Study the drawing (mm; zero at the part's minimum x, y, z) and answer. A direction names the side the tool comes from. Coordinates: 2 decimals unless noted, no trailing zeros. Order: outer loops, then holes, each group sorted by start corner. A loop starts at its lowest first (then second) coordinate and runs counter-clockwise, first axis right, second up. Notation, with made-up numbers: M 33.25,66 L 74.25,66 A12 ccw 74.25,79 Z; hole C 40,0 d9. An arc over 180 degrees is marked long. Use a Markdown table: item, result. Add a question column.
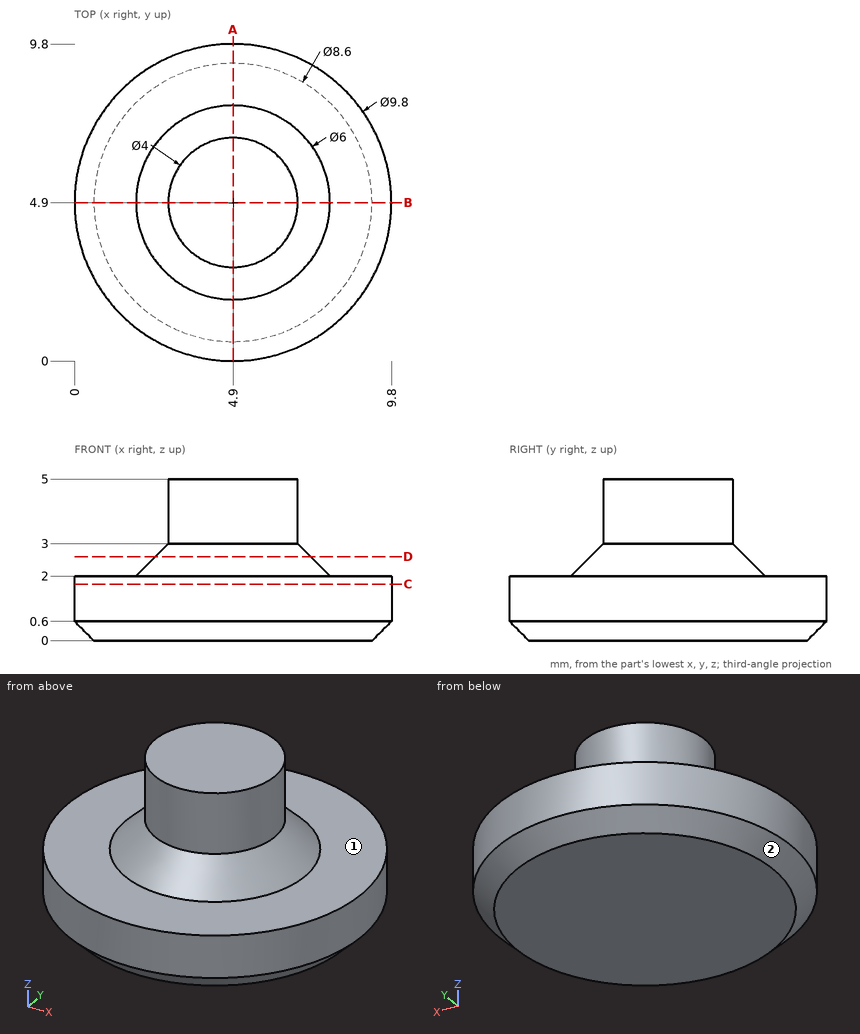
(1) A cutting plane is placed at D-D on z = 2.6. Write down the section's boundary in (x, y), plus the area to 3 significant figures.
(2) A cutting plane is placed at C-C on z = 1.75. Write down the section's boundary in (x, y), plus the area to 3 significant figures.
(3) Which of the six approach directions +Z, -Z, +X, -X, +Y, -Y give full straight-line access (tool end or side, diameter ignored) to the marked faces 1 and 2?
(4) Straight lines are drawn through the part: line 1 (Z direction, x = 8.75, y = 5.75); line 2 (X direction, y = 8.25, z = 1.2); line 3 (X direction, y = 5.75, z = 1.6). For each, find the intervals that lie inside material, in ascending order.
(5) A cutting plane is placed at A-A on x = 4.9. Write down the section's boundary in (y, z).
(6) Given P1, Ø3, axis at x = 3.5, z = 3, coming from the -Y side; P2, Ø1.5, axis at y = 1.5, z = 1.5, coming from the -X side; P3, Ø2, axis at x = 3.5, z = 4, coming from the -Y side, each flat-ended and moving along its own axis, determine where each tip first touches the part or whether it passes through.
From the geometry:
| question | item | result |
|---|---|---|
| 1 | outline | C 4.9,4.9 d4.8 |
| 1 | area | 18.1 mm2 |
| 2 | outline | C 4.9,4.9 d9.8 |
| 2 | area | 75.4 mm2 |
| 3 | face 1 | +Z |
| 3 | face 2 | -Z |
| 4 | line 1 | z = 0 to 2 |
| 4 | line 2 | x = 1.32 to 8.48 |
| 4 | line 3 | x = 0.07 to 9.73 |
| 5 | outline | M 0,0.6 L 0.6,0 L 9.2,0 L 9.8,0.6 L 9.8,2 L 7.9,2 L 6.9,3 L 6.9,5 L 2.9,5 L 2.9,3 L 1.9,2 L 0,2 Z |
| 6 | P1 | stops at y = 0.01 |
| 6 | P2 | stops at x = 0.78 |
| 6 | P3 | stops at y = 2.94 |
